Answer from the drawing. Dimensions are ordinates in mm from the lowest x, y and z of the part. Coordinates: 2 decimals unless noted, no trailing zeros. Write each loop counter-clockwise with the first axis right and the second up, starting at its lowest first coordinate (ties: lowest second). Pieces come first, ordered by that corner, then holes. Notation, with made-up numbers: M -8,61 L 34,61 A21 ccw 34,69 Z; hole C 46.25,80 d11. An arc over 180 degrees is marked long. Put each result on its own line as item: value. Start each with the question number.
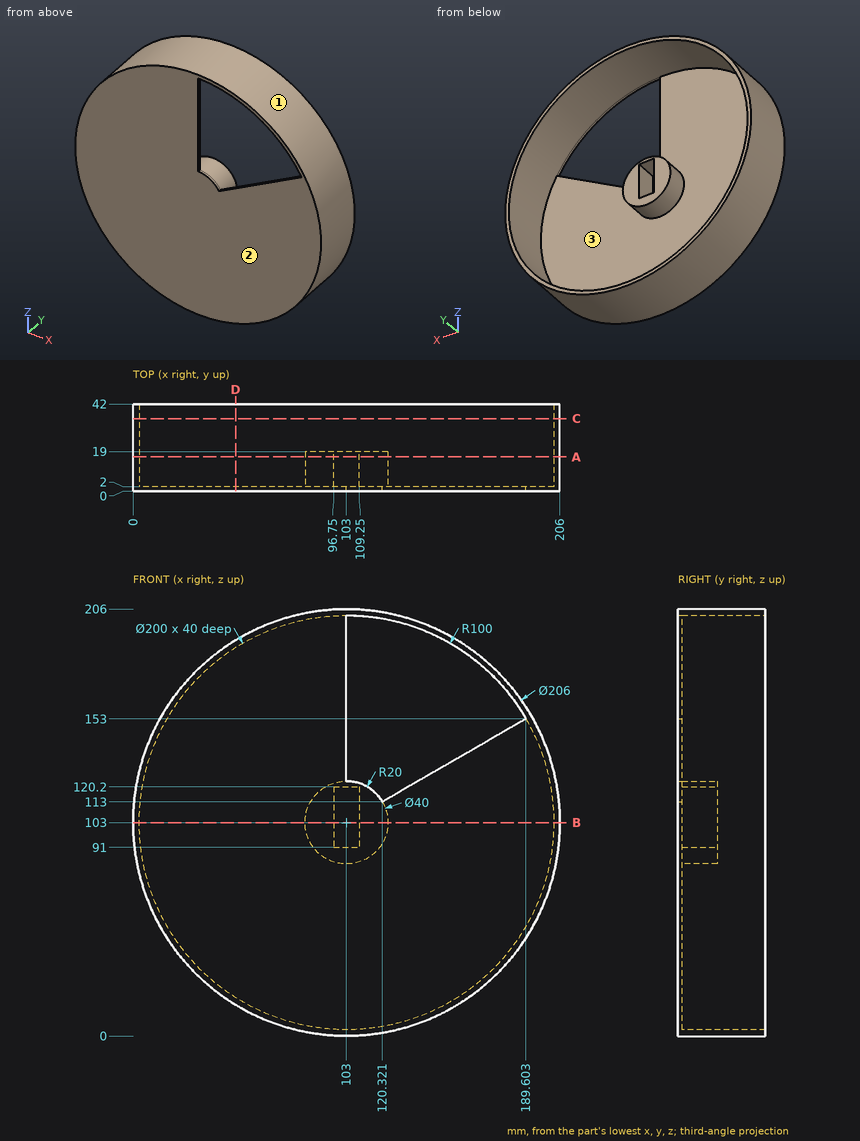
1) A cutting plane is placed at A-A on y = 16.5. Write down the section's boundary in (x, z).
2) Straight lines are drawn through the part: probe 1 along X at (y, z) = (17, 103); probe 2 along X at (y, z) = (24, 103); probe 3 along Y at (x, z) = (38, 120). For each, find the intervals that lie inside material, in ascending order.
3) A cutting plane is placed at D-D on x = 49.5. Write down the section's boundary in (y, z) (1 decimal).
4) A cutting plane is placed at B-B on z = 103. Write down the section's boundary in (x, y), then the cut area to 3 significant figures.
5) Determine the mould class of the marked faces 1, 2 and 3 for opening direction Z: +Z half, -Z half, draft (parallel to the pull), parting line (faces both ways), or undercut.
6) Given pin 1 Ø1 at (y, z) = (15, 105) entering from -X; pin 2 Ø5 at (y, z) = (12, 112) entering from +X (1 decimal); pin 3 Ø2 at (x, y) = (121, 10) entering from -Z; pin 4 Ø6 at (x, y) = (101.5, 8.5) entering from +Z, each flat-ended and moving along its own axis, determine where each tip first touches the part or whether it passes through.
7) A cutting plane is placed at C-C on y = 35. Write down the section's boundary in (x, z).
Answers follow:
1. outline: C 103,103 d206; C 103,103 d40; hole C 103,103 d200; hole M 96.75,91 L 109.25,91 L 109.25,120.2 L 96.75,120.2 Z
2. probe 1: x = 0 to 3, 83 to 96.75, 109.25 to 123, 203 to 206
2. probe 2: x = 0 to 3, 203 to 206
2. probe 3: y = 0 to 2
3. outline: M 0,15 L 42,15 L 42,18.5 L 2,18.5 L 2,187.5 L 42,187.5 L 42,191 L 0,191 Z
4. outline: M 0,0 L 206,0 L 206,42 L 203,42 L 203,2 L 123,2 L 123,19 L 109.25,19 L 109.25,2 L 96.75,2 L 96.75,19 L 83,19 L 83,2 L 3,2 L 3,42 L 0,42 Z
4. area: 1,120 mm²
5. face 1: parting line
5. face 2: draft
5. face 3: undercut
6. pin 1: stops at x = 0.01
6. pin 2: stops at x = 205.8
6. pin 3: stops at z = 1.41
6. pin 4: stops at z = 206
7. outline: C 103,103 d206; hole C 103,103 d200
